from build123d import *

# Parameters (mm, degrees)
SKETCH3_R          = 6
CUT_EXTRUDE2_DEPTH = 16
SKETCH4_R          = 8.5
CUT_EXTRUDE3_DEPTH = 10


with BuildPart() as part:
    # Sketch1 → Revolve1 (revolve)
    with BuildSketch(Plane.XY, mode=Mode.PRIVATE) as revolve1_sk:
        Polygon((-90.158227848, -16.376582278), (-100.158227848, -16.376582278), (-100.158227848, -2.376582278), (-55.158227848, -2.376582278), (-55.158227848, 20.123417722), (-40.158227848, 20.123417722), (-40.158227848, -8.876582278), (-90.158227848, -8.876582278), align=None)
    revolve(revolve1_sk.sketch.rotate(Axis((-100.158227848, -54.876582278, 0), (1, 0, 0)), 90), axis=Axis((-100.158227848, -54.876582278, 0), (1, 0, 0)))

    # Sketch3 → Cut-Extrude2 (cut)
    with BuildSketch(Plane(origin=(-40.158227848, 0, 0), x_dir=(0, 0, -1), z_dir=(1, 0, 0))):
        with Locations((45.254833996, -100.131416274)):
            Circle(SKETCH3_R)
        with Locations(Location((-45.254833996, -100.131416274, 0), (0, 0, 180))):
            Circle(SKETCH3_R)
    extrude(amount=-CUT_EXTRUDE2_DEPTH, mode=Mode.SUBTRACT)

    # Sketch4 → Cut-Extrude3 (cut)
    with BuildSketch(Plane(origin=(-40.158227848, 0, 0), x_dir=(0, 0, -1), z_dir=(1, 0, 0))):
        with Locations((-45.254833996, -100.131416274)):
            Circle(SKETCH4_R)
        with Locations((45.254833996, -100.131416274)):
            Circle(SKETCH4_R)
    extrude(amount=-CUT_EXTRUDE3_DEPTH, mode=Mode.SUBTRACT)


solid = part.part
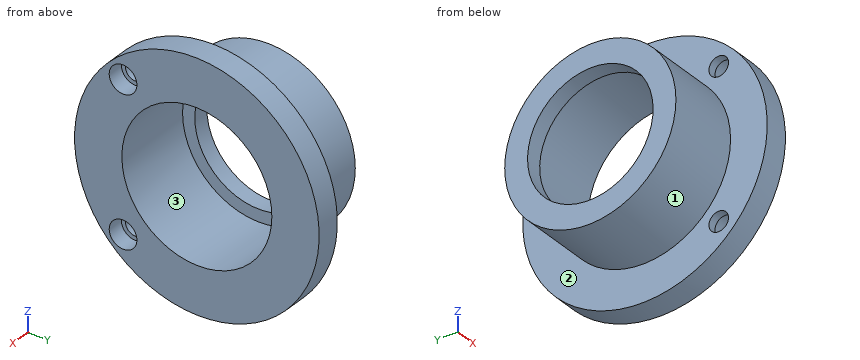
Input: part model. Units: mm. Frame: model coordinates. Face numbers are marked on the shaded views. Coordinates: 2 decimals unless noted, no trailing zeros. Loops run counter-clockwise (first coordinate to the right, second up) from the corner with the lowest first, then second, coordinate; pieces in that order, holes last. Notation, with made-up numbers: (3, 18) -> (27, 18) arc R30 cw to (27, 44) -> close; hole circle Ø11 at (-8, 67). An arc over 180 degrees is marked (long way). One line per item, written item: value.
(1) Draft query along Y for the marked faces 1, 2 and 3. Return one class per face: pulls with the +Y half, pulls with the -Y half, needs draft (parallel to the pull), parting line crosses it, or undercut.
Answer below:
face 1: parting line crosses it
face 2: needs draft
face 3: undercut
(2) Cut plane D-D (y = -13.5). Output: boundary loops of the cut face in (x, z).
Answer below:
outline: (-100.16, -32.31) -> (-55.16, -32.31) -> (-55.16, -62.55) -> (-40.16, -62.55) -> (-40.16, -20.1) -> (-90.16, -20.1) -> (-90.16, 20.1) -> (-40.16, 20.1) -> (-40.16, 62.55) -> (-55.16, 62.55) -> (-55.16, 32.31) -> (-100.16, 32.31) -> close
(3) Cut plane A-A (z = 0). Output: boundary loops of the cut face in (x, y).
Answer below:
outline: (-100.16, -107.38) -> (-55.16, -107.38) -> (-55.16, -129.88) -> (-40.16, -129.88) -> (-40.16, -100.88) -> (-90.16, -100.88) -> (-90.16, -93.38) -> (-100.16, -93.38) -> close; (-100.16, -16.38) -> (-90.16, -16.38) -> (-90.16, -8.88) -> (-40.16, -8.88) -> (-40.16, 20.12) -> (-55.16, 20.12) -> (-55.16, -2.38) -> (-100.16, -2.38) -> close
(4) Cut plane B-B (y = -35). Output: boundary loops of the cut face in (x, z).
Answer below:
outline: (-100.16, -48.59) -> (-55.16, -48.59) -> (-55.16, -72.32) -> (-40.16, -72.32) -> (-40.16, -41.48) -> (-90.16, -41.48) -> (-90.16, -32.97) -> (-100.16, -32.97) -> close; (-100.16, 32.97) -> (-90.16, 32.97) -> (-90.16, 41.48) -> (-40.16, 41.48) -> (-40.16, 72.32) -> (-55.16, 72.32) -> (-55.16, 48.59) -> (-100.16, 48.59) -> close
(5) Ray query, line 1 along Y through (x, z) = (-64, 0); line 2 along X through (y, z) = (-9, 40); line 3 along Z through (x, y) = (-95, -82). Return the intervals inside material, ascending.
Answer below:
line 1: y = -107.38 to -100.88, -8.88 to -2.38
line 2: x = -55.16 to -40.16
line 3: z = -44.95 to -27.32, 27.32 to 44.95
(6) Pin query (flat end, axial travel): pin 1 Ø6 at (x, z) = (-88, 51) entering from +Y; pin 2 Ø15.5 at (y, z) = (-100.13, 45.25) entering from -X; pin 3 Ø3 at (x, y) = (-93, -44) entering from +Z; pin 4 Ø18.5 at (y, z) = (-97.5, 43) entering from +X. Return the tip coordinate at first contact, or that it passes through.
Answer below:
pin 1: stops at y = -33.61
pin 2: stops at x = -55.16
pin 3: stops at z = 51.66
pin 4: stops at x = -40.16
(7) Cut plane C-C (x = -83). Output: boundary loops of the cut face in (y, z), then the cut area to 3 significant figures.
Answer below:
outline: circle Ø105 at (-54.88, 0); hole circle Ø92 at (-54.88, 0)
area: 2,010 mm2
